For this review, take the finished solid that the model builds, in its own axes (mm). A direction names the side the tool comes from. Coordinates: 2 decimals unless noted, no trailing zeros. Order: outer loops, then holes, each group sorted by start corner. A loop starts at its lowest first (then second) coordinate and runs counter-clockwise, first axis right, second up. Notation, with made-up numbers: (58.25, 24) -> (78.25, 24) arc R30 cw to (78.25, 59) -> close; hole circle Ø5 at (77.5, -8). An arc over 180 degrees is marked (long way). Write item = value, one per line. Start each with the question number.
1) Consider section A-A on y = 0. Give the boundary of the cut face in (x, z), and give its area (3 significant figures).
2) Wall thickness on probe 1 along X at (y, z) = (-1.5, 1.5); probe 2 along Y at (x, z) = (-23, 5.75); probe 3 along Y at (x, z) = (-10.5, 4.5): over which ranges is each line inside the solid? List them lowest first. Write a range as [from, to].
3) Draft analysis for pull direction X (two halves, no side actions). For faces 3 (the face through (34, 0, 5)), 4 (the face through (-34, 0, 5)), 5 (the face through (-24.45, 0.06, 5.07)), 6 (the face through (0, 10, 10)), state which applies: +X half, -X half, draft (parallel to the pull), parting line (faces both ways), or undercut.
4) Consider section B-B on x = 3. Give the boundary of the cut face in (y, z).
5) Consider section D-D on z = 7.25. Give the boundary of the cut face in (x, y), and give its area (3 significant figures).
6) Insertion check: pin 1 Ø3.5 at (x, y) = (-23, 0) entering from +Z. The pin has a flat end and moves straight along its axis. Give the tip position at first contact, or say it passes through.
7) Consider section C-C on y = -5.25. Give the boundary of the cut face in (x, z), and give its area (3 significant figures).
8) Machinability: for faces 1 (the face through (0, -15, 5)), 2 (the face through (0, 7.5, 5)), which of the approach directions +Z, -Z, +X, -X, +Y, -Y give a long, thin tool a straight path to every point of the face, cutting with its end or side? Answer none if there is none.
Autodesk Inventor part; units mm, degrees
ref_plane "YZ Plane" through (0, 0, 0) normal (1, 0, 0) x (0, 1, 0)
ref_plane "XZ Plane" through (0, 0, 0) normal (0, 1, 0) x (-1, 0, 0)
ref_plane "XY Plane" through (0, 0, 0) normal (0, 0, 1) x (1, 0, 0)
sketch "Sketch1" plane through (0, 0, 0) normal (0, 0, 1) x (1, 0, 0)
  line L0 (-34, 15) -> (34, 15)
  line L1 (34, 15) -> (34, -15)
  line L2 (34, -15) -> (-34, -15)
  line L3 (-34, -15) -> (-34, 15)
  line L4 (-34, 15) -> (34, -15) construction
  line L5 (34, 15) -> (-34, -15) construction
  point P0 (0, 0)
  dimension "d0" = 68
  dimension "d1" = 30
extrude "Extrusion1" add sketch "Sketch1" along normal blind 10
sketch "Sketch2" plane through (0, 0, 10) normal (0, 0, 1) x (1, 0, 0)
  line L0 (-14, 7.5) -> (14, 7.5)
  line L1 (14, 7.5) -> (14, -7.5)
  line L2 (14, -7.5) -> (-14, -7.5)
  line L3 (-14, -7.5) -> (-14, 7.5)
  line L4 (-14, 7.5) -> (14, -7.5) construction
  line L5 (14, 7.5) -> (-14, -7.5) construction
  point P0 (0, 0)
  dimension "d4" = 28
  dimension "d5" = 15
extrude "Extrusion2" cut sketch "Sketch2" against normal blind 10
sketch "Sketch3" plane through (0, 0, 10) normal (0, 0, 1) x (1, 0, 0)
  circle A0 centre (-23, 0) radius 1.4515
  circle A1 centre (23, 0) radius 1.4515
  line L0 (-14, -7.5) -> (-14, 7.5)
  line L1 (14, 7.5) -> (14, -7.5)
  point P0 (0, 0)
  dimension "d8" = 2.903
  dimension "d9" = 2.903
  dimension "d10" = 9
  dimension "d11" = 9
extrude "Extrusion3" cut sketch "Sketch3" against normal blind 10
properties part number "1st arm closing"
Answer sheet:
q1.outline = (-34, 0) -> (-24.45, 0) -> (-24.45, 10) -> (-34, 10) -> close; (-21.55, 0) -> (-14, 0) -> (-14, 10) -> (-21.55, 10) -> close; (14, 0) -> (21.55, 0) -> (21.55, 10) -> (14, 10) -> close; (24.45, 0) -> (34, 0) -> (34, 10) -> (24.45, 10) -> close
q1.area = 342 mm2
q2.probe_1 = [-34, -14], [14, 34]
q2.probe_2 = [-15, -1.45], [1.45, 15]
q2.probe_3 = [-15, -7.5], [7.5, 15]
q3.face_3 = +X half
q3.face_4 = -X half
q3.face_5 = undercut
q3.face_6 = draft
q4.outline = (-15, 0) -> (-7.5, 0) -> (-7.5, 10) -> (-15, 10) -> close; (7.5, 0) -> (15, 0) -> (15, 10) -> (7.5, 10) -> close
q5.outline = (-34, -15) -> (34, -15) -> (34, 15) -> (-34, 15) -> close; hole circle Ø2.9 at (-23, 0); hole (-14, -7.5) -> (14, -7.5) -> (14, 7.5) -> (-14, 7.5) -> close; hole circle Ø2.9 at (23, 0)
q5.area = 1,610 mm2
q6.pin_1 = 10
q7.outline = (-34, 0) -> (-14, 0) -> (-14, 10) -> (-34, 10) -> close; (14, 0) -> (34, 0) -> (34, 10) -> (14, 10) -> close
q7.area = 400 mm2
q8.face_1 = +Z, -Z, +X, -X, -Y
q8.face_2 = +Z, -Z
